Source: CAD feature listing. Evaluate the final solid. Frame: model axes, mm. A direction names the side the tool comes from. Round coordinates to 2 decimals unless told otherwise and drop trailing zeros. Order: outer loops, then holes, each group sorted by start corner. A loop starts at its lowest first (then second) coordinate and runs counter-clockwise, first axis right, second up. Notation, with made-up numbers: (79.5, -38) - (115.5, -38) arc R21 ccw to (115.5, -19) - close; hole circle Ø9 at (-25, 64.5). An arc over 180 degrees is marked (long way). Put each result on its own line as item: value. Start each with the question number.
1) Contact query for flat-ended pins moving along their axis: P1, Ø1, axis at x = -2, y = 5, coming from the -Z side; P2, Ø6, axis at x = -2, z = 22, coming from the +Y side; P3, Ø2, axis at y = 2.5, z = 7, coming from the +X side. Output: stop coordinate, or through.
2) Section A-A on z = 8.25. Output: boundary loops of the cut face in (x, y), then the cut area to 3 significant figures.
3) Mould query, pull axis Y, two halves, no side actions, for faces 4 (the face through (-2.476, 0.345, 1.282)), 5 (the face through (-2, -2, 0)), 6 (the face through (-0.86, -6.58, 3.99)). Classes: +Y half, -Y half, draft (parallel to the pull), parting line (faces both ways), or undercut.
4) Line query: probe 1 along X at (y, z) = (0, 3.5); probe 2 along Y at (x, z) = (0.75, 1.75); probe 3 along Z at (x, y) = (1.5, 1.25). Output: solid intervals per line, ascending. Write a range as [from, to].
5) Access query for faces 1 (the face through (0, 0, 24.4)), 2 (the face through (3, -3, 4.4)), 3 (the face through (-1.5, -2, 1.3)). Directions: +Z, -Z, +X, -X, +Y, -Y. A direction counts if a zero-diameter tool reaches every point of the face in a straight line with its end or side. Return the directions, or none.
Autodesk Inventor part; units mm, degrees
ref_plane "YZ Plane" through (0, 0, 0) normal (1, 0, 0) x (0, 1, 0)
ref_plane "XZ Plane" through (0, 0, 0) normal (0, 1, 0) x (-1, 0, 0)
ref_plane "XY Plane" through (0, 0, 0) normal (0, 0, 1) x (1, 0, 0)
sketch "Sketch1" plane through (0, 0, 0) normal (0, 0, 1) x (1, 0, 0)
  circle A0 centre (0, 0) radius 6.635
  circle A1 centre (0, 0) radius 4
  dimension "d0" = 13.27
  dimension "d1" = 8
extrude "Extrusion1" add sketch "Sketch1" along normal blind 4.4
extrude "Extrusion2" add sketch "Sketch1" along normal blind 24.4 contours A1
sketch "Boceto2" plane through (0, 0, 0) normal (0, 0, -1) x (-1, 0, 0)
  line L0 (2.2909, 1.7564) -> (2.6666, -1.1058)
  line L1 (2.6666, -1.1058) -> (0.3756, -2.8622)
  line L2 (0.3756, -2.8622) -> (-2.2909, -1.7564)
  line L3 (-2.2909, -1.7564) -> (-2.6666, 1.1058)
  line L4 (-2.6666, 1.1058) -> (-0.3756, 2.8622)
  line L5 (-0.3756, 2.8622) -> (2.2909, 1.7564)
  point P0 (0, 0)
  point P1 (0, 0)
  dimension "d6" = 5
extrude "Extrusión3" cut sketch "Boceto2" against normal blind 2.6
thread "Rosca1"
fillet "Empalme1" radius 3.6 1 edges at (-6.635, 0, 0)
chamfer "Chaflán2" distance 0.4 angle 45 1 edges at (-4, 0, 24.4)
properties part number "Tornillo allen cabeza boton M8x20mm"
Answer sheet:
1. P1: z = 0.51
1. P2: y = 4
1. P3: x = 3.71
2. outline: circle Ø8 at (0, 0)
2. area: 50.3 mm^2
3. face 4: undercut
3. face 5: draft
3. face 6: parting line
4. probe 1: [-6.63, 6.63]
4. probe 2: [-6.08, -2.4], [2.58, 6.08]
4. probe 3: [2.6, 24.4]
5. face 1: +Z, +X, -X, +Y, -Y
5. face 2: +Z
5. face 3: -Z
